Drawing for the job (mm, zero at the part's lowest x, y, z). Round coordinates to 2 decimals unless told otherwise and drop trailing zeros. Loops run counter-clockwise (first coordinate to the right, second up) from the corner with the lowest first, then second, coordinate; pieces in that order, holes last. Notation, with made-up numbers: (59.25, 81.5) -> (64.25, 81.5) arc R19 ccw to (64.25, 95.5) -> close; hole circle Ø9 at (55, 12.5). An arc over 180 degrees is marked (long way). Put each result on its own line as item: value. Start each with the question number.
Item 1: Drill centre lines: probe 1 along Y at (x, z) = (9, 30) (1 decimal); probe 2 along Y at (x, z) = (8.5, 9) (1 decimal); probe 3 along X at (y, z) = (32, 32.5) (1 decimal). Where is each one in solid material? Low to high. Write a range as [from, to].
Item 2: Pull direction Z, two halves, no side cores. Call the marked faces 1, 2 and 3: +Z half, -Z half, draft (parallel to the pull), parting line (faces both ways), or undercut.
Item 3: Flat gauge pin, fed straight in: pin 1 Ø2.5 at (x, y) = (4.76, 55.56) entering from -Z. Where does the tip first touch, or does it go through?
Item 4: Cut at C-C, the plane z = 11. List the corners of the cut face in (x, y) (1 decimal).
Item 5: Cut at A-A, the plane x = 50. List the corners of the cut face in (y, z) (1 decimal), plus the area to 3 significant figures.
Item 6: Cut at B-B, the plane y = 38.5. List the corners of the cut face in (x, z) (1 decimal), plus the area to 3 significant figures.
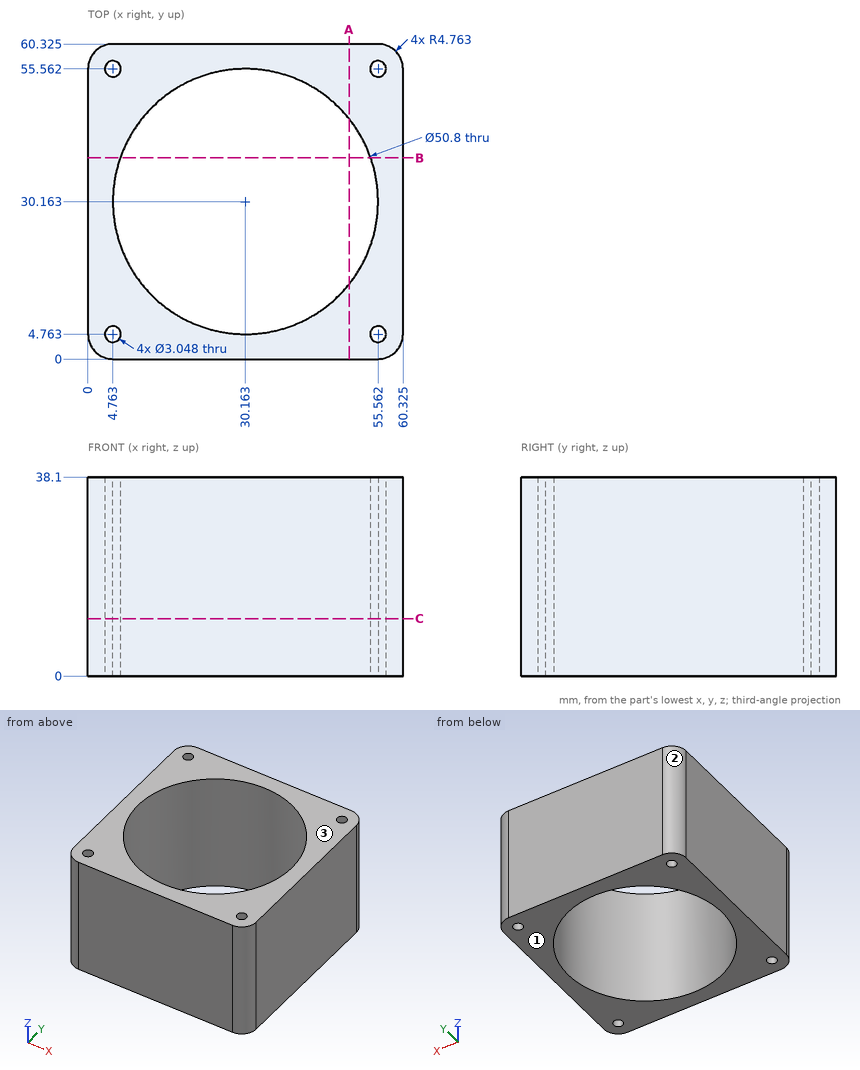
Reply:
1. probe 1: y = [0, 16.1], [44.2, 60.3]
1. probe 2: y = [0, 16.9], [43.4, 60.3]
1. probe 3: x = [0, 4.8], [55.5, 60.3]
2. face 1: -Z half
2. face 2: draft
2. face 3: +Z half
3. pin 1: passes through
4. outline: (0, 4.8) arc R4.8 ccw to (4.8, 0) -> (55.6, 0) arc R4.8 ccw to (60.3, 4.8) -> (60.3, 55.6) arc R4.8 ccw to (55.6, 60.3) -> (4.8, 60.3) arc R4.8 ccw to (0, 55.6) -> close; hole circle Ø3 at (4.8, 4.8); hole circle Ø3 at (4.8, 55.6); hole circle Ø50.8 at (30.2, 30.2); hole circle Ø3 at (55.6, 4.8); hole circle Ø3 at (55.6, 55.6)
5. outline: (0, 0) -> (14.3, 0) -> (14.3, 38.1) -> (0, 38.1) -> close; (46, 0) -> (60.3, 0) -> (60.3, 38.1) -> (46, 38.1) -> close
5. area: 1,090 mm^2
6. outline: (0, 0) -> (6.2, 0) -> (6.2, 38.1) -> (0, 38.1) -> close; (54.2, 0) -> (60.3, 0) -> (60.3, 38.1) -> (54.2, 38.1) -> close
6. area: 470 mm^2
